Input: part model. Units: mm. Frame: model coordinates. Give positions to 0.01 mm unless a question says otherwise; leave off trailing zeros. Loops run counter-clockwise (first coordinate to the right, second up) from the corner with the lowest first, then second, coordinate; pieces in that order, holes last. Notation, with made-up numbers: (55, -6.5) -> (113, -6.5) arc R36 ccw to (113, 29.5) -> close; hole circle Ø7 at (69.25, 44.25). An arc over 180 degrees is marked (long way). Answer as a JSON object with one key per item and string values. Group by question number.
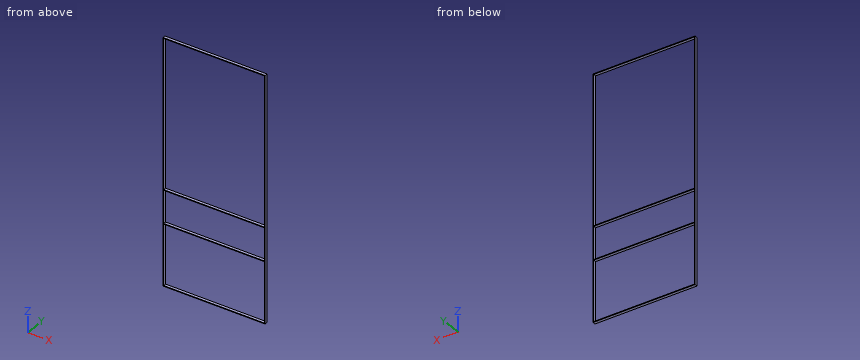
```python
from build123d import *

# Parameters (mm, degrees)
F0_W     = 750
F0_H     = 1800
F0_W_2   = 739.999995
F0_H_2   = 1789.999995
F1_DEPTH = 20
F2_W     = 748.980001
F2_H     = 5
F2_W_2   = 744.481355
F3_DEPTH = 20


with BuildPart() as f1:
    # F0 (on Front) → F1 (new body)
    with BuildSketch(Plane.XZ):
        with Locations((297.36115, 591.838682)):
            Rectangle(F0_W, F0_H)
        with Locations((297.361151, 591.838682)):
            Rectangle(F0_W_2, F0_H_2, mode=Mode.SUBTRACT)
    extrude(amount=F1_DEPTH)

    # F2 (on Front) → F3 (join)
    with BuildSketch(Plane.XZ):
        with Locations((297.594332, 389.002619)):
            Rectangle(F2_W, F2_H)
        with Locations((297.196076, 144.002619)):
            Rectangle(F2_W_2, F2_H)
    extrude(amount=F3_DEPTH)


solid = f1.part
```
Q1. Section A-A on x = 452. Return the cut outline in (y, z), then the cut area to 3 significant figures.
Q2. Section C-C on y = -5.5. Return the cut outline in (x, z), then the cut area to 3 significant figures.
Q3. Section B-B on z = 866.5. Return the cut outline in (x, y), then the cut area to 3 significant figures.
Q4. Ray query, probe 1 along Z at (x, y) = (641.5, -3.5); probe 2 along X at (y, z) = (-7.5, 787). Return the intervals inside material, ascending.
Numbers:
{
 "1": {"outline": "(-20, -308.16) -> (0, -308.16) -> (0, -303.16) -> (-20, -303.16) -> close; (-20, 141.5) -> (0, 141.5) -> (0, 146.5) -> (-20, 146.5) -> close; (-20, 386.5) -> (0, 386.5) -> (0, 391.5) -> (-20, 391.5) -> close; (-20, 1486.84) -> (0, 1486.84) -> (0, 1491.84) -> (-20, 1491.84) -> close", "area": "400 mm²"},
 "2": {"outline": "(-77.64, -308.16) -> (672.36, -308.16) -> (672.36, 1491.84) -> (-77.64, 1491.84) -> close; hole (-72.64, -303.16) -> (667.36, -303.16) -> (667.36, 141.5) -> (-72.64, 141.5) -> close; hole (-72.64, 146.5) -> (667.36, 146.5) -> (667.36, 386.5) -> (-72.64, 386.5) -> close; hole (-72.64, 391.5) -> (667.36, 391.5) -> (667.36, 1486.84) -> (-72.64, 1486.84) -> close", "area": "32,800 mm²"},
 "3": {"outline": "(-77.64, -20) -> (-72.64, -20) -> (-72.64, 0) -> (-77.64, 0) -> close; (667.36, -20) -> (672.36, -20) -> (672.36, 0) -> (667.36, 0) -> close", "area": "200 mm²"},
 "4": {"probe 1": "z = -308.16 to -303.16, 141.5 to 146.5, 386.5 to 391.5, 1486.84 to 1491.84", "probe 2": "x = -77.64 to -72.64, 667.36 to 672.36"}
}
